Answer from the drawing. Dimensions are ordinates in mm from the lowest x, y and z of the part. A direction names the side the tool comes from. Give positions to 0.01 mm unless a question says otherwise; leave off trailing zeros. Order: outer loops, then holes, each group sorted by start corner. A loop starts at its lowest first (then second) coordinate and runs counter-clockwise, first axis right, second up. Notation, with made-up numbers: (72, 44) -> (104, 44) arc R20 ccw to (104, 80) -> close; hole circle Ø7 at (21.5, 84). An arc over 180 degrees is marked (long way). Answer as CSV lines item,"result". Start each with the question number.
1) Find section C-C (y = 12.75). Determine the outline of the cut face in (x, z) (3 decimals), and give its area (3 significant figures).
2) Straight lines are drawn through the part: L1, parallel to Z at x = 10, y = 5; L2, parallel to X at y = 10.25, z = 12.5; L3, parallel to Z at x = 7.75, y = 0.5. For each, find the intervals that lie inside material, in ascending order. Write a range as from..to.
3) For the marked faces 1 and 2, determine the directions among +Z, -Z, +X, -X, +Y, -Y from which every point of the face is accessible in a straight line to the end or side of a thin tool.
4) Find section B-B (y = 1.75). Determine the outline of the cut face in (x, z).
5) Flat-ended cylindrical pins translate along their axes: pin 1 Ø4 at (x, z) = (9, 10.5) entering from +Y; pin 2 Ø3 at (x, y) = (5, 3) entering from +Z; pin 3 Ø2 at (y, z) = (10, 6) entering from +X; pin 4 Ø4 at (x, y) = (14.5, 12) entering from -Z. Find the tip coordinate at first contact, or state that the pin passes through.
6) Find section D-D (y = 9.25). Determine the outline of the cut face in (x, z).
7) Find section A-A (z = 8). Determine the outline of the cut face in (x, y).
8) The mould has two halves that part along Z. Classify the marked faces 3, 4, 5 and 6: +Z half, -Z half, draft (parallel to the pull), parting line (faces both ways), or undercut.
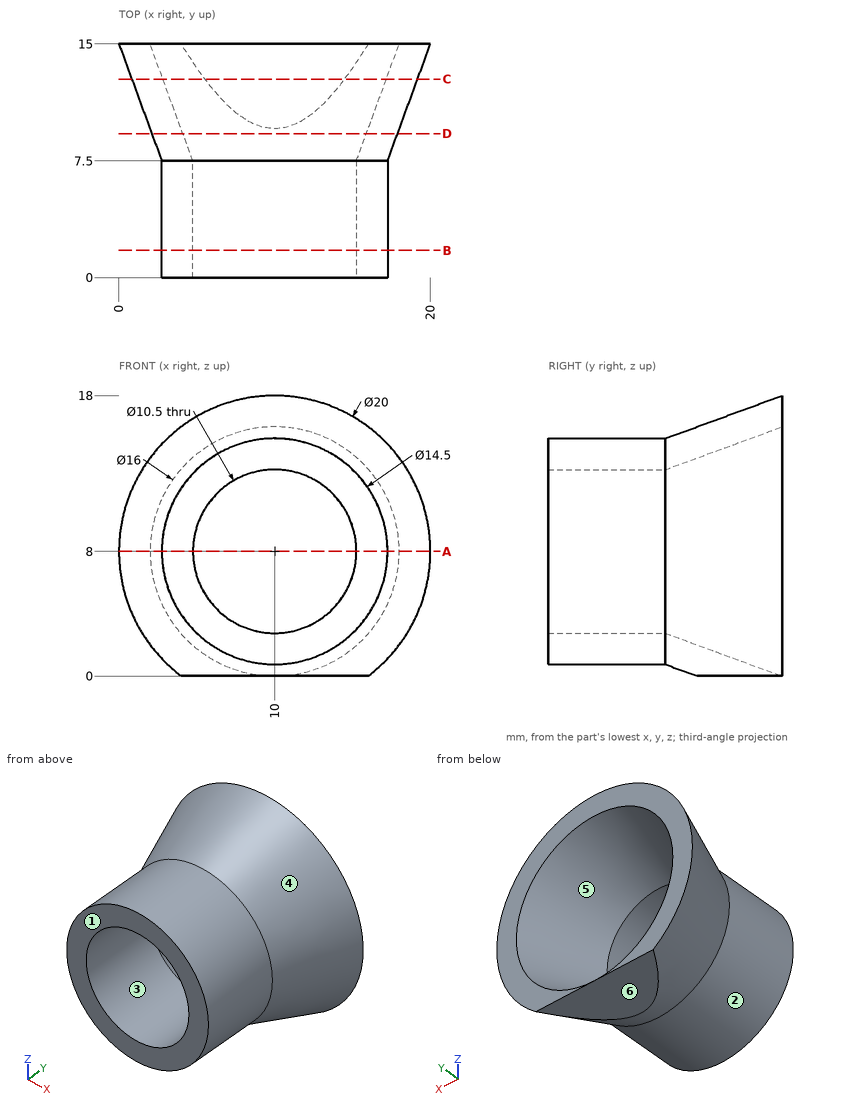
Findings below:
1,outline,"(5.508, 0) -> (14.492, 0) arc R9.175 ccw (long way) to start; hole circle Ø14.35 at (10, 8)"
1,area,"95.6 mm²"
2,L1,"0.75..2.75, 13.25..15.25"
2,L2,"3.08..5.65, 14.35..16.92"
2,L3,"1.11..3.26, 12.74..14.89"
3,face 1,"+Z, -Z, +X, -X, -Y"
3,face 2,"-Y"
4,outline,"circle Ø14.5 at (10, 8); hole circle Ø10.5 at (10, 8)"
5,pin 1,"through"
5,pin 2,"z = 14.35"
5,pin 3,"x = 18.35"
5,pin 4,"z = 0"
6,outline,"circle Ø15.78 at (10, 8); hole circle Ø11.78 at (10, 8)"
7,outline,"(0, 15) -> (2.75, 7.5) -> (2.75, 0) -> (4.75, 0) -> (4.75, 7.5) -> (2, 15) -> close; (15.25, 0) -> (17.25, 0) -> (17.25, 7.5) -> (20, 15) -> (18, 15) -> (15.25, 7.5) -> close"
8,face 3,"undercut"
8,face 4,"parting line"
8,face 5,"undercut"
8,face 6,"-Z half"
